from build123d import *

# Parameters (mm, degrees)
F1_DEPTH = 60.325
F2_DEPTH = 19.05
F0_W     = 19.05
F0_H     = 34.798
F3_DEPTH = 19.05
F4_DEPTH = 19.05
F8_R     = 6.35
F9_DEPTH = 25.4
F10_R    = 7.874
F11_R    = 5.08
F12_R    = 2.54


with BuildPart() as f1:
    # F0 (on Front) → F1 (new body)
    with BuildSketch(Plane.XZ):
        with BuildLine():
            ThreePointArc((-38.3635606445, 0), (-44.9103098714, -15.8052507731), (-60.7155606445, -22.352))
            Line((-60.7155606445, -22.352), (31.1308393555, -22.352))
            Line((31.1308393555, -22.352), (25.1364393555, 0))
            Line((25.1364393555, 0), (-38.3635606445, 0))
        make_face()
        Polygon((25.1364393555, 0), (31.1308393555, -22.352), (56.5308393555, -22.352), (56.5308393555, 0), align=None)
        Polygon((56.5308393555, 0), (56.5308393555, -22.352), (133.4928393555, -22.352), (133.4928393555, 0), (89.3730393555, 0), (70.3230393555, 0), align=None)
    extrude(amount=-F1_DEPTH)

    # F0 (on Front) → F2 (cut)
    with BuildSketch(Plane.XZ):
        Polygon((25.1364393555, 0), (31.1308393555, -22.352), (56.5308393555, -22.352), (56.5308393555, 0), align=None)
    extrude(amount=-F2_DEPTH, mode=Mode.SUBTRACT)

    # F0 (on Front) → F3 (join)
    with BuildSketch(Plane.XZ):
        with BuildLine():
            ThreePointArc((70.3230393555, 34.798), (66.7492677026, 16.0821939471), (56.5308393555, 0))
            Line((56.5308393555, 0), (70.3230393555, 0))
            Line((70.3230393555, 0), (70.3230393555, 34.798))
        make_face()
        with Locations((79.8480393555, 17.399)):
            Rectangle(F0_W, F0_H)
    extrude(amount=-F3_DEPTH)


with BuildPart() as f4:
    # F0 (on Front) → F4 (new body)
    with BuildSketch(Plane.XZ):
        with BuildLine():
            ThreePointArc((-38.3635606445, 0), (-76.5208114176, 15.8052507731), (-60.7155606445, -22.352))
            ThreePointArc((-60.7155606445, -22.352), (-44.9103098714, -15.8052507731), (-38.3635606445, 0))
        make_face()
        with BuildLine():
            ThreePointArc((-60.7155606445, -12.7), (-69.6958167656, 8.9802561211), (-48.0155606445, 0))
            ThreePointArc((-48.0155606445, 0), (-51.7353045234, -8.9802561211), (-60.7155606445, -12.7))
        make_face(mode=Mode.SUBTRACT)
    extrude(amount=-F4_DEPTH)


with BuildPart() as f6_1:
    # F6: instance of F4
    add(f4.part.mirror(Plane.XZ.offset(-30.1625)))


with BuildPart() as f1_1:
    add(f1.part)

    # F7: union F4, F6_1
    add(f4.part)
    add(f6_1.part)

    # F8 (on face) → F9 (cut)
    with BuildSketch(Plane.XY):
        with Locations((94.6308393555, 37.973)):
            Circle(F8_R)
    extrude(amount=-F9_DEPTH, mode=Mode.SUBTRACT)

    # F10
    f10_edges = [f1_1.edges().sort_by_distance(p)[0] for p in [
        (133.492839, 30.1625, 0),
    ]]
    fillet(f10_edges, radius=F10_R)

    # F11
    f11_edges = [f1_1.edges().sort_by_distance(p)[0] for p in [
        (89.373039, 9.525, 34.798),
    ]]
    fillet(f11_edges, radius=F11_R)

    # F12
    f12_edges = [f1_1.edges().sort_by_distance(p)[0] for p in [
        (-38.363561, 50.8, 0),
        (-38.363561, 9.525, 0),
        (89.373039, 9.525, 0),
    ]]
    fillet(f12_edges, radius=F12_R)


solid = f1_1.part
Read the model definition and answer for the solid it produces. Units are mm, in the model's axes. A direction names the side the tool comes from. Round coordinates to 2 decimals unless told otherwise and drop trailing zeros. Write each loop counter-clockwise with the first axis right and the second up, starting at its lowest first coordinate (ties: lowest second). Pieces come first, ordered by that corner, then holes. Notation, with made-up numbers: (38, 61.25) - (62, 61.25) arc R21 cw to (62, 98.25) - close; hole circle Ø9 at (19.5, 6.25). An arc over 180 degrees is marked (long way). Use a Markdown table: item, result.
(1) The part is cut by section A-A (y = 11). Write down the section's boundary in (x, z), then the cut area to 3 significant figures.
Reported:
| item | result |
|---|---|
| outline | (-60.72, -22.35) - (31.13, -22.35) - (25.14, 0) - (-35.95, 0) arc R2.54 cw to (-38.48, 2.28) arc R22.35 ccw (long way) to start; (56.53, -22.35) - (133.49, -22.35) - (133.49, -7.87) arc R7.87 ccw to (125.62, 0) - (91.91, 0) arc R2.54 cw to (89.37, 2.54) - (89.37, 29.72) arc R5.08 ccw to (84.29, 34.8) - (70.32, 34.8) arc R50.79 cw to (56.53, 0) - close; hole circle Ø25.4 at (-60.72, 0) |
| area | 5,170 mm2 |
(2) The part is cut by section D-D (y = 29). Write down the section's boundary in (x, z).
Reported:
| item | result |
|---|---|
| outline | (-60.72, -22.35) - (133.49, -22.35) - (133.49, -7.87) arc R7.87 ccw to (125.62, 0) - (-38.36, 0) arc R22.35 cw to start |
(3) The part is cut by section B-B (y = 50.5). Write down the section's boundary in (x, z).
Reported:
| item | result |
|---|---|
| outline | (-60.72, -22.35) - (133.49, -22.35) - (133.49, -7.87) arc R7.87 ccw to (125.62, 0) - (-35.95, 0) arc R2.54 cw to (-38.48, 2.28) arc R22.35 ccw (long way) to start; hole circle Ø25.4 at (-60.72, 0) |
(4) Which of the six approach directions +Z, -Z, +X, -X, +Y, -Y give full straight-line access (tool end or side, diameter ignored) to faces 1 (the flat face through (86, 0, 0)), 2 (the flat face through (28.09, 9.39, -11.02)), 3 (the flat face through (56.531, 9, -11)), 4 (the flat face through (78, 19.05, 18))?
Reported:
| item | result |
|---|---|
| face 1 | +Z, -Z, +X, -X, -Y |
| face 2 | +Z, -Y |
| face 3 | +Z, -Z, -Y |
| face 4 | +Z, +X, -X, +Y |
(5) Each of these flat-tipped pins is pushed along its axis until it touches: pin 1 Ø23 at (x, z) = (-60.72, 0) entering from -Y; pin 2 Ø12 at (y, z) = (48, 21) entering from -X; pin 3 Ø15 at (y, z) = (12.5, 13) entering from +X; pin 4 Ø21 at (y, z) = (8.5, -16) entering from -X. Where does it stop, or does it pass through?
Reported:
| item | result |
|---|---|
| pin 1 | through |
| pin 2 | x = -77.29 |
| pin 3 | x = 89.37 |
| pin 4 | x = -82.38 |
(6) The mould has two halves that part along Y. Classify faces 5 (the cylindrical face through (-76.82, 9.39, 15.5)), 6 (the flat face through (-70, 19.05, -10)), 7 (the flat face through (41, 19.05, -11)), 8 (the flat face through (-70, 41.275, -10)): released by +Y, released by -Y, zero draft, split by the parting line, or undercut.
Reported:
| item | result |
|---|---|
| face 5 | zero draft |
| face 6 | undercut |
| face 7 | released by -Y |
| face 8 | undercut |
(7) The part is cut by section C-C (x = -45). Write down the section's boundary in (y, z) (3 decimals), then the cut area to 3 significant figures.
Reported:
| item | result |
|---|---|
| outline | (0, -22.352) - (60.325, -22.352) - (60.325, 15.894) - (41.275, 15.894) - (41.275, -15.894) - (19.05, -15.894) - (19.05, 15.894) - (0, 15.894) - close |
| area | 1,600 mm2 |
(8) Straight lines are drawn through the part: line 1 along Z through (x, y) = (-61.5, 5.5); line 2 along X through (y, z) = (3, 8); line 3 along Y through (x, z) = (-58.5, 16) (3 decimals). For each, find the intervals that lie inside material, in ascending order. Write a range as [from, to].
Reported:
| item | result |
|---|---|
| line 1 | [-22.34, -12.68], [12.68, 22.34] |
| line 2 | [-81.59, -70.58], [-50.85, -39.84], [62.68, 89.37] |
| line 3 | [0, 19.05], [41.275, 60.325] |
